Could you check a few things on this model? Use its own coordinates, in mm. Face numbers are marked on the shaded views. Give positions to 0.01 mm unless a question says otherwise; leave off trailing zeros. Write each loop counter-clockwise with the first axis right and the second up, starting at its lowest first coordinate (ties: lowest second). Pieces come first, ordered by that corner, then holes. Notation, with made-up numbers: (32.25, 5) -> (62.25, 5) arc R23 ccw to (62.25, 32) -> close; hole circle Ø9 at (76, 45.5). An arc over 180 degrees is marked (long way). One line per question, with ' | ' between items.
from build123d import *

# Parameters (mm, degrees)
EXTRUDE_1_DEPTH = 60
FILLET_1_R      = 0.2


with BuildPart() as part:
    # 草图1 → 凸台-拉伸1 (new body)
    with BuildSketch(Plane.XY):
        with BuildLine():
            Line((-10, 0), (10, 0))
            ThreePointArc((10, 0), (11.767766953, -0.732233047), (12.5, -2.5))
            Line((12.5, -2.5), (12.5, -12.5))
            Line((12.5, -12.5), (11.9, -12.5))
            Line((11.9, -12.5), (11.9, -11.1))
            ThreePointArc((11.9, -11.1), (11.3, -10.5), (10.7, -11.1))
            Line((10.7, -11.1), (10.7, -12.5))
            Line((10.7, -12.5), (10.1, -12.5))
            Line((10.1, -12.5), (10.1, -5.5))
            Line((10.1, -5.5), (9, -5.5))
            Line((9, -5.5), (9, -3.866025404))
            ThreePointArc((9, -3.866025404), (10.366025404, -2.5), (8.5, -3))
            ThreePointArc((8.5, -3), (8.534074174, -3.258819045), (8.633974596, -3.5))
            Line((8.633974596, -3.5), (7, -3.5))
            Line((7, -3.5), (7, -2.4))
            Line((7, -2.4), (6.4, -2.4))
            Line((6.4, -2.4), (6.4, -1))
            Line((6.4, -1), (4.6, -1))
            Line((4.6, -1), (4.6, -2.4))
            Line((4.6, -2.4), (-4.6, -2.4))
            Line((-4.6, -2.4), (-4.6, -1))
            Line((-4.6, -1), (-6.4, -1))
            Line((-6.4, -1), (-6.4, -2.4))
            Line((-6.4, -2.4), (-7, -2.4))
            Line((-7, -2.4), (-7, -3.5))
            Line((-7, -3.5), (-8.633974596, -3.5))
            ThreePointArc((-8.633974596, -3.5), (-8.534074174, -3.258819045), (-8.5, -3))
            ThreePointArc((-8.5, -3), (-10.366025404, -2.5), (-9, -3.866025404))
            Line((-9, -3.866025404), (-9, -5.5))
            Line((-9, -5.5), (-10.1, -5.5))
            Line((-10.1, -5.5), (-10.1, -12.5))
            Line((-10.1, -12.5), (-10.8, -12.5))
            Line((-10.8, -12.5), (-10.8, -13.9))
            ThreePointArc((-10.8, -13.9), (-11.3, -14.4), (-11.8, -13.9))
            Line((-11.8, -13.9), (-11.8, -12.5))
            Line((-11.8, -12.5), (-12.5, -12.5))
            Line((-12.5, -12.5), (-12.5, -2.5))
            ThreePointArc((-12.5, -2.5), (-11.767766953, -0.732233047), (-10, 0))
        make_face()
    extrude(amount=EXTRUDE_1_DEPTH)

    # 圆角1
    fillet_1_edges = [part.edges().sort_by_distance(p)[0] for p in [
        (9, -3.866025404, 30),
        (8.633974596, -3.5, 30),
        (7, -3.5, 30),
        (7, -2.4, 30),
        (6.4, -2.4, 30),
        (-6.4, -2.4, 30),
        (-7, -2.4, 30),
        (-7, -3.5, 30),
        (-8.633974596, -3.5, 30),
        (-9, -3.866025404, 30),
    ]]
    fillet(fillet_1_edges, radius=FILLET_1_R)


solid = part.part
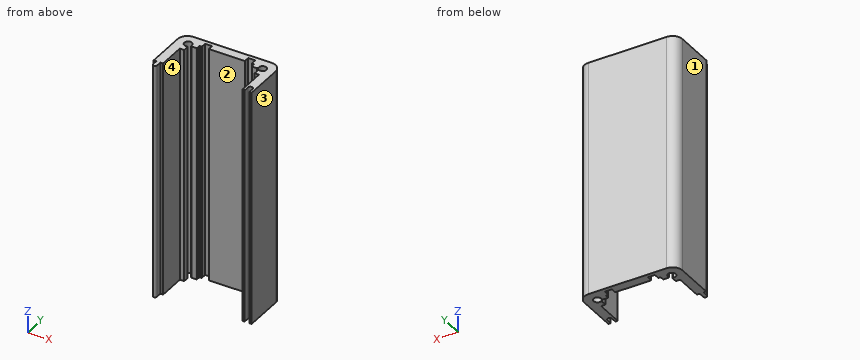
Q1. If we mould it in two halves opening along X, with no side actions, what happens to the marked faces 1, 2, 3 and 4? For each: +X half, -X half, draft (parallel to the pull), parting line (faces both ways), or undercut.
Answer below:
face 1: -X half | face 2: undercut | face 3: +X half | face 4: undercut
Q2. Imagine slicing it at B-B on x = 1.5. Please give me the cut outline in (y, z).
Answer below:
outline: (-2.4, 0) -> (0, 0) -> (0, 60) -> (-2.4, 60) -> close
Q3. If I drill on line 1 along X through (y, z) = (-3, 15); line 2 along Y through (x, z) = (9.5, 17.5); line 3 along X through (y, z) = (-2.5, 25.5), over which ranges is the centre line in solid material (lowest first)?
Answer below:
line 1: x = -12.5 to -10.5, -8.5 to -7, 7 to 8.5, 10.5 to 12.5 | line 2: y = -5.5 to -4, -2 to 0 | line 3: x = -12.5 to -10.37, -8.63 to -6.97, 6.97 to 8.63, 10.37 to 12.5
Q4. Will these pins go through, and if not, where does the flat tip stop? pin 1 (1.3 mm diameter, centred on y = -1.5, z = 23.5, fed in from +X); pin 2 (7.5 mm diameter, centred on x = 0.5, z = 40, fed in from -Y); pin 3 (0.6 mm diameter, centred on x = -7.5, z = 30, fed in from -Y).
Answer below:
pin 1: stops at x = 12.48 | pin 2: stops at y = -2.4 | pin 3: stops at y = -3.5
Q5. Imagine slicing it at A-A on y = -6.5. Please give me the cut outline in (x, z).
Answer below:
outline: (-12.5, 0) -> (-10.1, 0) -> (-10.1, 60) -> (-12.5, 60) -> close; (10.1, 0) -> (12.5, 0) -> (12.5, 60) -> (10.1, 60) -> close
